from build123d import *

# Parameters (mm, degrees)
SKETCH_1_W          = 86
SKETCH_1_H          = 44.4
EXTRUDE_1_DEPTH     = 19.6
EXTRUDE_2_DEPTH     = 5
SKETCH_3_W          = 26.733333333
SKETCH_3_H          = 42
SKETCH_3_W_2        = 27.333333334
CUT_EXTRUDE_1_DEPTH = 18.4
FILLET_1_R          = 3
EXTRUDE_3_DEPTH     = 0.2


with BuildPart() as part:
    # Эскиз1 → Бобышка-Вытянуть1 (new body)
    with BuildSketch(Plane.XY):
        Rectangle(SKETCH_1_W, SKETCH_1_H)
    extrude(amount=EXTRUDE_1_DEPTH)

    # Эскиз2 → Бобышка-Вытянуть2 (add)
    with BuildSketch(Plane.XY):
        with BuildLine():
            Line((43, 17.2), (43, 13.108775687))
            ThreePointArc((43, 13.108775687), (53.273546839, 0), (43, -13.108775687))
            Line((43, -13.108775687), (43, -17.2))
            ThreePointArc((43, -17.2), (57.273546839, 0), (43, 17.2))
        make_face()
    extrude(amount=EXTRUDE_2_DEPTH)

    # Эскиз3 → Вырез-Вытянуть1 (cut)
    with BuildSketch(Plane.XY.offset(19.6)):
        with Locations((-28.033333334, 0)):
            Rectangle(SKETCH_3_W, SKETCH_3_H)
        with Locations((0.2, 0)):
            Rectangle(SKETCH_3_W_2, SKETCH_3_H)
        with Locations((28.433333334, 0)):
            Rectangle(SKETCH_3_W, SKETCH_3_H)
    extrude(amount=-CUT_EXTRUDE_1_DEPTH, mode=Mode.SUBTRACT)

    # Скругление1
    fillet_1_edges = [part.edges().sort_by_distance(p)[0] for p in [
        (-41.4, 21, 10.4),
        (-41.4, -21, 10.4),
        (-43, -22.2, 9.8),
        (-43, 22.2, 9.8),
    ]]
    fillet(fillet_1_edges, radius=FILLET_1_R)

    # Эскиз4 → Бобышка-Вытянуть3 (add)
    with BuildSketch(Plane(origin=(0, 0, 0), x_dir=(-1, 0, 0), z_dir=(0, 0, -1))):
        with BuildLine():
            Line((-50.772048757, 13.611868188), (-27.989807175, 22.2))
            ThreePointArc((-27.989807175, 22.2), (-43.674993872, 29.297054885), (-50.772048757, 13.611868188))
        make_face()
        with BuildLine():
            Line((-50.772048757, -13.611868188), (-27.989807175, -22.2))
            ThreePointArc((-27.989807175, -22.2), (-43.674993872, -29.297054885), (-50.772048757, -13.611868188))
        make_face()
        with BuildLine():
            Line((43, 9.068731744), (28.793502644, 22.2))
            ThreePointArc((28.793502644, 22.2), (46.369205759, 26.964337461), (43, 9.068731744))
        make_face()
        with BuildLine():
            Line((43, -9.068731744), (28.793502644, -22.2))
            ThreePointArc((28.793502644, -22.2), (46.369205759, -26.964337461), (43, -9.068731744))
        make_face()
    extrude(amount=-EXTRUDE_3_DEPTH)


solid = part.part
CAD build for the part. Positions are in the model's coordinates, mm. A direction names the side the tool comes from. Round coordinates to 2 decimals unless told otherwise and drop trailing zeros. Write each loop counter-clockwise with the first axis right and the second up, starting at its lowest first coordinate (ties: lowest second). Pieces come first, ordered by that corner, then holes. Notation, with made-up numbers: (-32.5, 56) -> (-26.5, 56) arc R30 cw to (-26.5, 92) -> close; hole circle Ø8 at (-7.5, 11). An arc over 180 degrees is marked (long way). Answer as a JSON object with one key per item and string values.
(1) Band-saw the part on A-A, the plane z = 16. List the corners of the cut face in (x, y), then the cut area to 3 significant figures.
Reported:
{"outline": "(-43, -19.2) arc R3 ccw to (-40, -22.2) -> (43, -22.2) -> (43, 22.2) -> (-40, 22.2) arc R3 ccw to (-43, 19.2) -> close; hole (-41.4, -18) arc R3 ccw to (-38.4, -21) -> (-14.67, -21) -> (-14.67, 21) -> (-38.4, 21) arc R3 ccw to (-41.4, 18) -> close; hole (-13.47, -21) -> (13.87, -21) -> (13.87, 21) -> (-13.47, 21) -> close; hole (15.07, -21) -> (41.8, -21) -> (41.8, 21) -> (15.07, 21) -> close", "area": "425 mm^2"}
(2) Band-saw the part on B-B, the plane y = -1. List the corners of the cut face in (x, z).
Reported:
{"outline": "(-43, 0) -> (43, 0) -> (43, 19.6) -> (41.8, 19.6) -> (41.8, 1.2) -> (15.07, 1.2) -> (15.07, 19.6) -> (13.87, 19.6) -> (13.87, 1.2) -> (-13.47, 1.2) -> (-13.47, 19.6) -> (-14.67, 19.6) -> (-14.67, 1.2) -> (-41.4, 1.2) -> (-41.4, 19.6) -> (-43, 19.6) -> close; (53.24, 0) -> (57.24, 0) -> (57.24, 5) -> (53.24, 5) -> close"}
(3) Probe probe 1 along X at (y, z) = (12.5, 6.5); probe 2 along Y at (x, z) = (-8.5, 11.5); probe 3 along X at (y, z) = (-7, 4). List the from-to ranges inside material, lowest first. Write a range as [from, to].
Reported:
{"probe 1": "x = [-43, -41.4], [-14.67, -13.47], [13.87, 15.07], [41.8, 43]", "probe 2": "y = [-22.2, -21], [21, 22.2]", "probe 3": "x = [-43, -41.4], [-14.67, -13.47], [13.87, 15.07], [41.8, 43], [51.32, 55.81]"}
(4) Band-saw the part on C-C, the plane x = 2.5. List the corners of the cut face in (y, z), then the cut area to 3 significant figures.
Reported:
{"outline": "(-22.2, 0) -> (22.2, 0) -> (22.2, 19.6) -> (21, 19.6) -> (21, 1.2) -> (-21, 1.2) -> (-21, 19.6) -> (-22.2, 19.6) -> close", "area": "97.4 mm^2"}
(5) Which spindle directions (+Z, -Z, +X, -X, +Y, -Y) get a long thin tool onto all of the face, cutting with end or side? Do faces 1 (the face through (57.27, -0.34, 2.46)), 2 (the face through (3, 0, 0)), 3 (the face through (-28, 0, 1.2)). Say none if no direction does.
Reported:
{"face 1": "+Z, +X", "face 2": "-Z, +X, -X, +Y, -Y", "face 3": "+Z"}
(6) Two-plate mould, pull along Y, no slides. Class faces 4 (the face through (-42, 22, 0.2)), 5 (the face through (13.867, 0, 11)): +Y half, -Y half, draft (parallel to the pull), parting line (faces both ways), or undercut.
Reported:
{"face 4": "draft", "face 5": "undercut"}
(7) Pin check, flat tips, straight feed: P1, Ø8, axis at y = 15, z = 5, coming from the +X side; P2, Ø9, axis at x = -27.5, z = 15, coming from the +Y side; P3, Ø5, axis at y = 23, z = 9, coming from the +X side. Stop position of each tip, or through.
Reported:
{"P1": "stops at x = 53.38", "P2": "stops at y = 22.2", "P3": "stops at x = 43"}
(8) Band-saw the part on D-D, the plane x = 47. List the corners of the cut face in (y, z).
Reported:
{"outline": "(-27.4, 0) -> (-11.4, 0) -> (-11.4, 5) -> (-15.94, 5) -> (-15.94, 0.2) -> (-27.4, 0.2) -> close; (11.4, 0) -> (27.4, 0) -> (27.4, 0.2) -> (15.94, 0.2) -> (15.94, 5) -> (11.4, 5) -> close"}
